Geometry check sheet. Reference: the model listing, model coordinates, mm. A direction names the side the tool comes from. Coordinates: 2 decimals unless noted, no trailing zeros. Loops run counter-clockwise (first coordinate to the right, second up) from the corner with the lowest first, then second, coordinate; pieces in that order, holes last.
Autodesk Inventor part; units mm, degrees
ref_plane "YZ Plane" through (0, 0, 0) normal (1, 0, 0) x (0, 1, 0)
ref_plane "XZ Plane" through (0, 0, 0) normal (0, 1, 0) x (-1, 0, 0)
ref_plane "XY Plane" through (0, 0, 0) normal (0, 0, 1) x (1, 0, 0)
sketch "Sketch1" plane through (0, 0, 0) normal (0, 1, 0) x (-1, 0, 0)
  line L0 (44.45, 22.225) -> (-44.45, 22.225)
  line L1 (-44.45, 22.225) -> (-44.45, -22.225)
  line L2 (-44.45, -22.225) -> (44.45, -22.225)
  line L3 (44.45, -22.225) -> (44.45, 22.225)
  line L4 (44.45, 22.225) -> (-44.45, -22.225) construction
  line L5 (-44.45, 22.225) -> (44.45, -22.225) construction
  line L6 (0, 0) -> (-44.45, 0) construction
  line L7 (44.45, 28.575) -> (-57.15, 28.575)
  line L8 (-57.15, 28.575) -> (-57.15, -28.575)
  line L9 (-57.15, -28.575) -> (44.45, -28.575)
  line L10 (44.45, -28.575) -> (44.45, 28.575)
  line L11 (44.45, 28.575) -> (-57.15, -28.575) construction
  line L12 (-57.15, 28.575) -> (44.45, -28.575) construction
  point P0 (-6.35, 0)
  point P1 (44.45, 22.225)
  dimension "d0" = 88.9
  dimension "d1" = 44.45
  dimension "d2" = 6.35
  dimension "d3" = 12.7
extrude "Extrusion1" add sketch "Sketch1" along normal blind 9.525 contours L0 L1 L2 L10 L9 L8 L7
chamfer "Chamfer1" distance 6.35 angle 45 4 edges at (44.45, 4.7625, 22.225) (57.15, 4.7625, 28.575) (44.45, 4.7625, -22.225) (57.15, 4.7625, -28.575)
fillet "Fillet1" radius 3.175 8 edges at (38.1, 4.7625, 22.225) (44.45, 4.7625, 15.875) (44.45, 4.7625, -15.875) (38.1, 4.7625, -22.225) (50.8, 4.7625, -28.575) (57.15, 4.7625, -22.225) (57.15, 4.7625, 22.225) (50.8, 4.7625, 28.575)
sketch "Sketch2" plane through (57.15, 0, 20.9099) normal (1, 0, 0) x (0, 0, -1)
  line L0 (35.4697, 9.525) -> (6.35, 9.525)
  line L1 (20.9099, 9.525) -> (20.9099, 0) construction
  line L2 (35.4697, 0) -> (6.35, 0)
  circle A0 centre (20.9099, 4.7625) radius 3.175 construction
  circle A1 centre (20.9099, 11.1125) radius 3.175
  line L3 (20.9099, 17.1125) -> (20.9099, 5.1125) construction
  line L4 (19.4099, 17.1125) -> (19.4099, 5.1125)
  line L5 (22.4099, 5.1125) -> (22.4099, 17.1125)
  arc A2 (22.4099, 17.1125) -> (19.4099, 17.1125) centre (20.9099, 17.1125) ccw
  arc A3 (19.4099, 5.1125) -> (22.4099, 5.1125) centre (20.9099, 5.1125) ccw
  point P0 (18.1602, 9.525)
  point P1 (23.6595, 9.525)
  point P2 (22.4099, 8.3142)
  point P3 (19.4099, 8.3142)
  dimension "d10" = 6.35
  dimension "d20" = 6.35
  dimension "d21" = 6.35
  dimension "d22" = 3
  dimension "d23" = 12
sketch "Sketch4" plane through (0, 9.525, 0) normal (0, 1, 0) x (1, 0, 0)
  line L0 (44.45, 14.5599) -> (44.45, -14.5599)
  line L1 (44.45, 0) -> (57.15, 0) construction
  line L2 (57.15, -20.9099) -> (57.15, 20.9099)
  line L3 (47.625, -9.525) -> (53.975, -9.525) construction
  line L4 (53.975, -9.525) -> (53.975, 9.525) construction
  line L5 (53.975, 9.525) -> (47.625, 9.525) construction
  line L6 (47.625, 9.525) -> (47.625, -9.525) construction
  line L7 (47.625, -9.525) -> (53.975, 9.525) construction
  line L8 (53.975, -9.525) -> (47.625, 9.525) construction
  circle A0 centre (47.625, -9.525) radius 1.5
  circle A1 centre (47.625, 9.525) radius 1.5
  circle A2 centre (53.975, -9.525) radius 1.5
  circle A3 centre (53.975, 9.525) radius 1.5
  point P0 (0, 0)
  point P1 (50.8, 0)
  dimension "d27" = 6.35
  dimension "d28" = 19.05
  dimension "d29" = 3
  dimension "d32" = 19.05
  dimension "d35" = 6.35
extrude "Extrusion5" cut sketch "Sketch4" against normal through all
chamfer "Chamfer2" distance 3.175 angle 45 2 edges at (-44.45, 9.525, -25.4) (-44.45, 9.525, 25.4)
equation "\"d32\" = d28"
equation "\"d35\" = d27"
properties part number "Rack" material "Aluminum 6061"
(1) Sectioned sample at A-A on x = 0.5. Record the cut outline in (y, z) (3 decimals), and give its area (3 significant figures).
Findings:
outline: (0, -28.575) - (9.525, -28.575) - (9.525, -22.225) - (0, -22.225) - close; (0, 22.225) - (9.525, 22.225) - (9.525, 28.575) - (0, 28.575) - close
area: 121 mm2
(2) Gauge pin test, flat end, axial feed: pin 1 Ø1.8 at (x, z) = (47.625, -9.525) entering from -Y. Record the tip position at first contact, or that the pin passes through.
Findings:
pin 1: passes through
(3) Access from +Z, -Z, +X, -X, +Y, -Y to the whole of each face (thin tool, end or side, straight path). Record for faces 1 (the cylindrical face through (56.915, 4.829, -22.109)), 2 (the cylindrical face through (44.215, 4.829, -15.759)).
Findings:
face 1: -Z, +X, +Y, -Y
face 2: -X, +Y, -Y
(4) Draft check along Z on faces 3 (the cylindrical face through (56.9, 4.83, 22.14)), 4 (the flat face through (57.15, 5, 0)), 5 (the flat face through (41.306, 4.829, 19.019)). Enter one of: +Z half, -Z half, draft (parallel to the pull), parting line (faces both ways), or undercut.
Findings:
face 3: +Z half
face 4: draft
face 5: undercut
(5) Sectioned sample at C-C on z = -1.5. Record the cut outline in (x, y) (3 decimals).
Findings:
outline: (44.45, 0) - (57.15, 0) - (57.15, 9.525) - (44.45, 9.525) - close
(6) Sectioned sample at D-D on x = 40.5. Record the cut outline in (y, z) (3 decimals).
Findings:
outline: (0, -28.575) - (9.525, -28.575) - (9.525, -19.825) - (0, -19.825) - close; (0, 19.825) - (9.525, 19.825) - (9.525, 28.575) - (0, 28.575) - close
(7) Scan lines: L1, parallel to Z at x = 26.5, y = 7.25 (3 decimals); L2, parallel to X at y = 5.5, z = 9; L3, parallel to X at y = 5.75, z = -13. Record each from-to range of solid material in increasing order.
Findings:
L1: z = -28.575 to -22.225, 22.225 to 28.575
L2: x = 44.45 to 46.22, 49.03 to 52.57, 55.38 to 57.15
L3: x = 44.45 to 57.15
(8) Sectioned sample at B-B on y = 7.5. Record the cut outline in (x, z) (3 decimals).
Findings:
outline: (-43.3, -28.575) - (49.485, -28.575) arc R3.175 ccw to (51.73, -27.645) - (56.22, -23.155) arc R3.175 ccw to (57.15, -20.91) - (57.15, 20.91) arc R3.175 ccw to (56.22, 23.155) - (51.73, 27.645) arc R3.175 ccw to (49.485, 28.575) - (-43.3, 28.575) - (-43.3, 22.225) - (36.785, 22.225) arc R3.175 cw to (39.03, 21.295) - (43.52, 16.805) arc R3.175 cw to (44.45, 14.56) - (44.45, -14.56) arc R3.175 cw to (43.52, -16.805) - (39.03, -21.295) arc R3.175 cw to (36.785, -22.225) - (-43.3, -22.225) - close; hole circle Ø3 at (47.625, -9.525); hole circle Ø3 at (47.625, 9.525); hole circle Ø3 at (53.975, -9.525); hole circle Ø3 at (53.975, 9.525)
